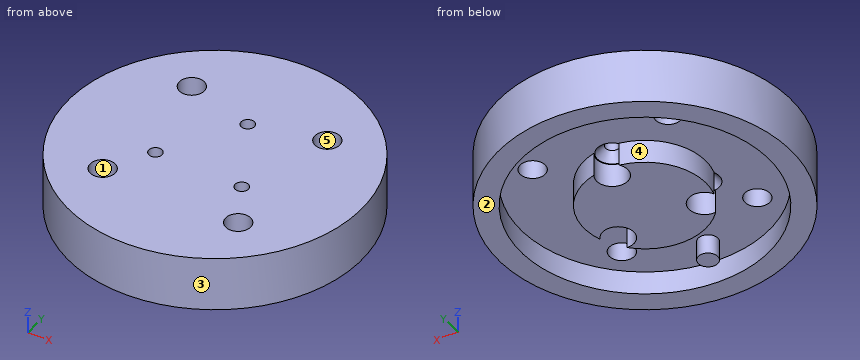
from build123d import *

# Parameters (mm, degrees)
SKETCH_R        = 37.5
SKETCH_R_2      = 1.7
SKETCH_R_3      = 3.2
PAD_DEPTH       = 8
SKETCH001_R     = 37.5
SKETCH001_R_2   = 31.8
PAD001_DEPTH    = 6
SKETCH002_R     = 2.5
PAD002_DEPTH    = 5
SKETCH003_R     = 15.6
PAD003_DEPTH    = 6
SKETCH004_R     = 4
POCKET_DEPTH    = 6
CHAMFER_SIZE    = 2.1
CHAMFER001_SIZE = 2.1
CHAMFER002_SIZE = 2.1


with BuildPart() as part:
    # Sketch → Pad (new body)
    with BuildSketch(Plane.XY):
        Circle(SKETCH_R)
        with Locations((-11.25833, -6.5)):
            Circle(SKETCH_R_2, mode=Mode.SUBTRACT)
        with Locations((11.25833, -6.5)):
            Circle(SKETCH_R_2, mode=Mode.SUBTRACT)
        with Locations((0, 13)):
            Circle(SKETCH_R_2, mode=Mode.SUBTRACT)
        with Locations((-17.67767, 17.67767)):
            Circle(SKETCH_R_3, mode=Mode.SUBTRACT)
        with Locations((17.67767, 17.67767)):
            Circle(SKETCH_R_3, mode=Mode.SUBTRACT)
        with Locations((-17.67767, -17.67767)):
            Circle(SKETCH_R_3, mode=Mode.SUBTRACT)
        with Locations((17.67767, -17.67767)):
            Circle(SKETCH_R_3, mode=Mode.SUBTRACT)
    extrude(amount=PAD_DEPTH)

    # Sketch001 → Pad001 (new body)
    with BuildSketch(Plane(origin=(0, 0, 0), x_dir=(1, 0, 0), z_dir=(0, 0, -1))):
        Circle(SKETCH001_R)
        Circle(SKETCH001_R_2, mode=Mode.SUBTRACT)
    extrude(amount=PAD001_DEPTH)

    # Sketch002 → Pad002 (new body)
    with BuildSketch(Plane(origin=(0, 0, 0), x_dir=(1, 0, 0), z_dir=(0, 0, -1))):
        with Locations((0, 25)):
            Circle(SKETCH002_R)
    extrude(amount=PAD002_DEPTH)

    # Sketch003 → Pad003 (new body)
    with BuildSketch(Plane(origin=(0, 0, 0), x_dir=(1, 0, 0), z_dir=(0, 0, -1))):
        Circle(SKETCH003_R)
    extrude(amount=PAD003_DEPTH)

    # Sketch004 → Pocket (cut)
    with BuildSketch(Plane(origin=(0, 0, -6), x_dir=(1, 0, 0), z_dir=(0, 0, -1))):
        with Locations((-11.25833, 6.5)):
            Circle(SKETCH004_R)
        with Locations((11.25833, 6.5)):
            Circle(SKETCH004_R)
        with Locations((0, -13)):
            Circle(SKETCH004_R)
    extrude(amount=-POCKET_DEPTH, mode=Mode.SUBTRACT)

    # Chamfer
    chamfer_edges = [part.edges().sort_by_distance(p)[0] for p in [
        (9.55833, -6.5, 0),
    ]]
    chamfer(chamfer_edges, length=CHAMFER_SIZE)

    # Chamfer001
    chamfer001_edges = [part.edges().sort_by_distance(p)[0] for p in [
        (-12.95833, -6.5, 0),
    ]]
    chamfer(chamfer001_edges, length=CHAMFER001_SIZE)

    # Chamfer002
    chamfer002_edges = [part.edges().sort_by_distance(p)[0] for p in [
        (-1.7, 13, 0),
    ]]
    chamfer(chamfer002_edges, length=CHAMFER002_SIZE)


solid = part.part
The model under review builds one solid part; all positions refer to its coordinate system, in mm. Face numbers are marked on the shaded views. A direction names the side the tool comes from. Give positions to 0.01 mm unless a question says otherwise; leave off trailing zeros. Loops run counter-clockwise (first coordinate to the right, second up) from the corner with the lowest first, then second, coordinate; pieces in that order, holes last. Notation, with made-up numbers: (32, 86.5) -> (37, 86.5) arc R9 cw to (37, 101.5) -> close; hole circle Ø7 at (76.5, 13.5). An arc over 180 degrees is marked (long way). Write each question's results on one line, items separated by ' | '.
1) Draft analysis for pull direction X (two halves, no side actions). For the marked faces 1, 2 and 3, state which applies: pulls with the +X half, pulls with the -X half, needs draft (parallel to the pull), parting line crosses it, or undercut.
Conclusion:
face 1: undercut | face 2: needs draft | face 3: parting line crosses it
2) Take a section at B-B, the plane x = 0. Give the boundary of the cut face in (y, z), plus the area to 3 significant figures.
Conclusion:
outline: (-37.5, -6) -> (-31.8, -6) -> (-31.8, 0) -> (-27.5, 0) -> (-27.5, -5) -> (-22.5, -5) -> (-22.5, 0) -> (-15.6, 0) -> (-15.6, -6) -> (9, -6) -> (9, 0) -> (9.2, 0) -> (11.3, 2.1) -> (11.3, 8) -> (-37.5, 8) -> close; (14.7, 2.1) -> (16.8, 0) -> (31.8, 0) -> (31.8, -6) -> (37.5, -6) -> (37.5, 8) -> (14.7, 8) -> close | area: 809 mm^2
3) For line 1 along X through (y, z) = (-19.5, 3.75); line 2 along Y through (x, z) = (-15, 5.25); line 3 along Y through (x, z) = (-9.5, -2), list the stretches that pass through material, from the lowest coordinate up. Write a range as from..to.
Conclusion:
line 1: x = -32.03..-20.31, -15.05..15.05, 20.31..32.03 | line 2: y = -34.37..-19.43, -15.93..15.93, 19.43..34.37 | line 3: y = -36.28..-30.35, -12.37..-10.09, -2.91..12.37, 30.35..36.28
4) Take a section at D-D, the plane x = 18. Give the boundary of the cut face in (y, z).
Conclusion:
outline: (-32.9, -6) -> (-26.22, -6) -> (-26.22, 0) -> (-20.86, 0) -> (-20.86, 8) -> (-32.9, 8) -> close; (-14.49, 0) -> (14.49, 0) -> (14.49, 8) -> (-14.49, 8) -> close; (20.86, 0) -> (26.22, 0) -> (26.22, -6) -> (32.9, -6) -> (32.9, 8) -> (20.86, 8) -> close
5) Take a section at C-C, the plane y = -6.5. Give the boundary of the cut face in (x, z), plus the area to 3 significant figures.
Conclusion:
outline: (-36.93, -6) -> (-31.13, -6) -> (-31.13, 0) -> (-15.06, 0) -> (-12.96, 2.1) -> (-12.96, 8) -> (-36.93, 8) -> close; (-9.56, 2.1) -> (-7.46, 0) -> (-7.26, 0) -> (-7.26, -6) -> (7.26, -6) -> (7.26, 0) -> (7.46, 0) -> (9.56, 2.1) -> (9.56, 8) -> (-9.56, 8) -> close; (12.96, 2.1) -> (15.06, 0) -> (31.13, 0) -> (31.13, -6) -> (36.93, -6) -> (36.93, 8) -> (12.96, 8) -> close | area: 684 mm^2
6) Insertion check: pin 1 Ø2 at (x, y) = (-11.26, -6.5) entering from -Z; pin 2 Ø13 at (x, y) = (-11.26, -6.5) entering from +Z; pin 3 Ø1.5 at (y, z) = (-26.5, 6.5) entering from -X; pin 4 Ø6 at (y, z) = (-8, 3) entering from -X. Each pin has a flat end and moves straight along its axis. Give the tip position at first contact, or say it passes through.
Conclusion:
pin 1: passes through | pin 2: stops at z = 8 | pin 3: stops at x = -27.26 | pin 4: stops at x = -37.17
7) Tool access review of the marked faces 4 and 5: name each direction out of +Z, -Z, +X, -X, +Y, -Y from which nothing blocks a thin tool from reaching the whole face with its end or side.
Conclusion:
face 4: -Z | face 5: +Z, -Z
8) Take a section at A-A, the plane z = -2.5. Give the boundary of the cut face in (x, y), plus the area to 3 significant figures.
Conclusion:
outline: circle Ø75 at (0, 0); (-14.86, -4.76) arc R4 cw (long way) to (-11.55, -10.49) arc R15.6 ccw to (11.55, -10.49) arc R4 cw (long way) to (14.86, -4.76) arc R15.6 ccw to (3.31, 15.24) arc R4 cw (long way) to (-3.31, 15.24) arc R15.6 ccw to start; circle Ø5 at (0, -25); hole circle Ø63.6 at (0, 0) | area: 1,890 mm^2
